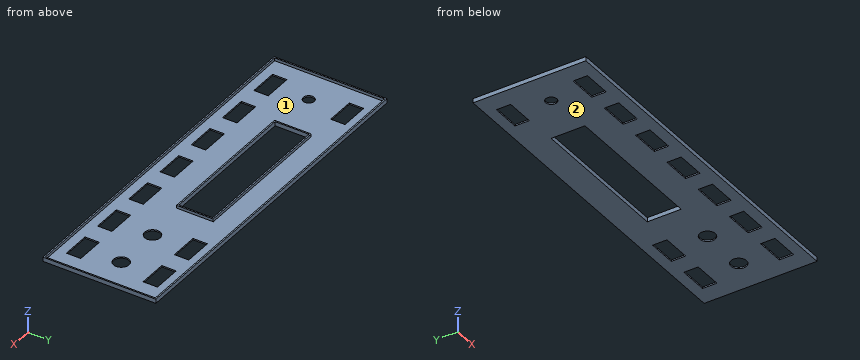
```python
from build123d import *

# Parameters (mm, degrees)
F0_W     = 158.75
F0_H     = 50.8
F0_W_2   = 12.827
F0_H_2   = 6.477
F0_W_3   = 66.04
F0_H_3   = 15.24
F1_DEPTH = 0.635
F2_D     = 6.985
F3_D     = 6.985
F5_W     = 158.75
F5_H     = 50.8
F5_W_2   = 157.48
F5_H_2   = 49.53
F6_DEPTH = 1.27
F7_W     = 67.31
F7_H     = 16.51
F7_W_2   = 66.04
F7_H_2   = 15.24
F8_DEPTH = 1.27
F9_D     = 4.953


with BuildPart() as f1:
    # F0 (on Top) → F1 (new body)
    with BuildSketch(Plane.XY):
        Rectangle(F0_W, F0_H)
        with Locations((-64.389, -17.272)):
            Rectangle(F0_W_2, F0_H_2, mode=Mode.SUBTRACT)
        with Locations((-42.926, -17.272)):
            Rectangle(F0_W_2, F0_H_2, mode=Mode.SUBTRACT)
        with Locations((-21.463, -17.272)):
            Rectangle(F0_W_2, F0_H_2, mode=Mode.SUBTRACT)
        with Locations((0, -17.272)):
            Rectangle(F0_W_2, F0_H_2, mode=Mode.SUBTRACT)
        with Locations((21.463, -17.272)):
            Rectangle(F0_W_2, F0_H_2, mode=Mode.SUBTRACT)
        with Locations((42.926, -17.272)):
            Rectangle(F0_W_2, F0_H_2, mode=Mode.SUBTRACT)
        with Locations((64.389, -17.272)):
            Rectangle(F0_W_2, F0_H_2, mode=Mode.SUBTRACT)
        with Locations((-10.541, 6.096)):
            Rectangle(F0_W_3, F0_H_3, mode=Mode.SUBTRACT)
        with Locations((-64.3255, 17.3355)):
            Rectangle(F0_W_2, F0_H_2, mode=Mode.SUBTRACT)
        with Locations((42.926, 17.272)):
            Rectangle(F0_W_2, F0_H_2, mode=Mode.SUBTRACT)
        with Locations((64.389, 17.272)):
            Rectangle(F0_W_2, F0_H_2, mode=Mode.SUBTRACT)
    extrude(amount=F1_DEPTH)

    # F2 (through all)
    with Locations(Plane(origin=(0, 0, 0), x_dir=(1, 0, 0), z_dir=(0, 0, -1))):
        with Locations((42.926, 0)):
            Hole(F2_D / 2)

    # F3 (through all)
    with Locations(Plane(origin=(0, 0, 0), x_dir=(1, 0, 0), z_dir=(0, 0, -1))):
        with Locations((64.389, 0)):
            Hole(F3_D / 2)

    # F5 (on offset) → F6 (join)
    with BuildSketch(Plane.XY.offset(0.635)):
        Rectangle(F5_W, F5_H)
        Rectangle(F5_W_2, F5_H_2, mode=Mode.SUBTRACT)
    extrude(amount=F6_DEPTH)

    # F7 (on offset) → F8 (join)
    with BuildSketch(Plane.XY.offset(0.635)):
        with Locations((-10.541, 6.096)):
            Rectangle(F7_W, F7_H)
        with Locations((-10.541, 6.096)):
            Rectangle(F7_W_2, F7_H_2, mode=Mode.SUBTRACT)
    extrude(amount=F8_DEPTH)

    # F9 (through all)
    with Locations(Plane(origin=(0, 0, 0), x_dir=(1, 0, 0), z_dir=(0, 0, -1))):
        with Locations((-64.389, 0)):
            Hole(F9_D / 2)


solid = f1.part
```
Model file for the job. Use its own axes, mm. Face numbers are marked on the shaded views. Coordinates: 2 decimals unless noted, no trailing zeros. Write each loop counter-clockwise with the first axis right and the second up, starting at its lowest first coordinate (ties: lowest second). Pieces come first, ordered by that corner, then holes. Notation, with made-up numbers: (82.5, -17) - (100.5, -17) arc R18 ccw to (100.5, 2) - close; hole circle Ø3 at (-1.5, 88.5). An arc over 180 degrees is marked (long way). Use a Markdown table: item, result. Add a question column.
Item 1: Drop a flat-ended pin along its axis: pin 1 (6 mm diameter, centred on x = 19, y = -11.5, fed in from +Z) (3 decimals). Give the stop position or say it passes through.
Item 2: Band-saw the part on C-C, the plane y = 0. Write the cut outline in (x, z) (1 decimal).
Item 3: Two-plate mould, pull along X, no slides. Class the marked faces 1 and 2: pulls with the +X half, pulls with the -X half, needs draft (parallel to the pull), parting line crosses it, or undercut.
Item 4: Band-saw the part on B-B, the plane x = 3. Write the cut outline in (y, z) (1 decimal), and give its area (3 significant figures).
Item 5: Drill centre lines: line 1 along X through (y, z) = (8, 1.05) (3 decimals); line 2 along Y through (x, z) = (-13.5, 1.55) (3 decimals); line 3 along X through (y, z) = (-20.5, 0.95) (3 decimals). Where is each one in solid material? Low to high.
Item 6: Band-saw the part on D-D, the plane x = -13.5. Write the cut outline in (y, z) (3 decimals), and give its area (3 significant figures).
Item 7: Band-saw the part on A-A, the plane z = 1.05. Write the cut outline in (x, y) (3 decimals).
A:
| question | item | result |
|---|---|---|
| 1 | pin 1 | stops at z = 0.635 |
| 2 | outline | (-79.4, 0) - (-66.9, 0) - (-66.9, 0.6) - (-78.7, 0.6) - (-78.7, 1.9) - (-79.4, 1.9) - close; (-61.9, 0) - (-43.6, 0) - (-43.6, 1.9) - (-44.2, 1.9) - (-44.2, 0.6) - (-61.9, 0.6) - close; (22.5, 0) - (39.4, 0) - (39.4, 0.6) - (23.1, 0.6) - (23.1, 1.9) - (22.5, 1.9) - close; (46.4, 0) - (60.9, 0) - (60.9, 0.6) - (46.4, 0.6) - close; (67.9, 0) - (79.4, 0) - (79.4, 1.9) - (78.7, 1.9) - (78.7, 0.6) - (67.9, 0.6) - close |
| 3 | face 1 | undercut |
| 3 | face 2 | needs draft |
| 4 | outline | (-25.4, 0) - (-20.5, 0) - (-20.5, 0.6) - (-24.8, 0.6) - (-24.8, 1.9) - (-25.4, 1.9) - close; (-14, 0) - (-1.5, 0) - (-1.5, 1.9) - (-2.2, 1.9) - (-2.2, 0.6) - (-14, 0.6) - close; (13.7, 0) - (25.4, 0) - (25.4, 1.9) - (24.8, 1.9) - (24.8, 0.6) - (14.4, 0.6) - (14.4, 1.9) - (13.7, 1.9) - close |
| 4 | area | 21.7 mm² |
| 5 | line 1 | x = -79.375 to -78.74, -44.196 to -43.561, 22.479 to 23.114, 78.74 to 79.375 |
| 5 | line 2 | y = -25.4 to -24.765, -2.159 to -1.524, 13.716 to 14.351, 24.765 to 25.4 |
| 5 | line 3 | x = -79.375 to -78.74, 78.74 to 79.375 |
| 6 | outline | (-25.4, 0) - (-1.524, 0) - (-1.524, 1.905) - (-2.159, 1.905) - (-2.159, 0.635) - (-24.765, 0.635) - (-24.765, 1.905) - (-25.4, 1.905) - close; (13.716, 0) - (25.4, 0) - (25.4, 1.905) - (24.765, 1.905) - (24.765, 0.635) - (14.351, 0.635) - (14.351, 1.905) - (13.716, 1.905) - close |
| 6 | area | 25.8 mm² |
| 7 | outline | (-79.375, -25.4) - (79.375, -25.4) - (79.375, 25.4) - (-79.375, 25.4) - close; (-44.196, -2.159) - (23.114, -2.159) - (23.114, 14.351) - (-44.196, 14.351) - close; hole (-78.74, -24.765) - (78.74, -24.765) - (78.74, 24.765) - (-78.74, 24.765) - close; hole (-43.561, -1.524) - (22.479, -1.524) - (22.479, 13.716) - (-43.561, 13.716) - close |
